Geometry check sheet. Reference: the model listing, model coordinates, mm. A direction names the side the tool comes from. Give positions to 0.01 mm unless a question says otherwise; leave off trailing zeros. Order: outer loops, then holes, each group sorted by start corner. A loop starts at its lowest first (then second) coordinate and runs counter-clockwise, first axis right, second up. Notation, with made-up numbers: M 51.5,30 L 78.5,30 A19 ccw 78.5,58 Z; hole C -25,6 d6. An arc over 180 degrees is marked long. Put each result on its own line as item: value. Start each with the question number.
Q1. Section check B-B on z = 16. Record the cut outline in (x, y).
Q2. Go/stop test with flat-tipped pins: pin 1 (7 mm diameter, centred on x = -13.5, y = 13, fed in from -Z); pin 2 (3.5 mm diameter, centred on y = 2, z = 36, fed in from -X); pin 3 (8 mm diameter, centred on y = 8, z = 33.5, fed in from +X); pin 4 (3.5 mm diameter, centred on x = 14, y = 2.5, fed in from +Z). Record where each tip stops, or that it passes through.
Q3. Material ranges on L1, parallel to X at y = 13.75, z = 18; L2, parallel to X at y = 2.5, z = 0; L3, parallel to Y at x = -19.76, z = 36.15, recorded low to high.
Q4. Access from +Z, -Z, +X, -X, +Y, -Y to the whole of each face (thin tool, end or side, straight path). Record for faces 1 (the flat face through (-25, 10, 15)), 2 (the flat face through (28, 3, 3)), 3 (the flat face through (45.296, 10.972, 37.535)), 4 (the flat face through (49, 11, 35)).
Q5. Section check A-A on x = 14. Record the cut outline in (y, z).
Q6. Section check C-C on z = -8.5. Record the cut outline in (x, y), then the cut area to 3 significant figures.
Q7. Section check D-D on y = 3.5. Record the cut outline in (x, z), then the cut area to 3 significant figures.
Q8. Mould release check, pull along Z, two halves, no side actions. Record for faces 5 (the cylindrical face through (-2.85, 3.45, 11.99)), 6 (the cylindrical face through (24.956, 3.451, -1.438)), 7 (the cylindrical face through (33.82, 3.45, 25.01)): +Z half, -Z half, draft (parallel to the pull), parting line (faces both ways), or undercut.
```python
from build123d import *

# Parameters (mm, degrees)
SKETCH1_R           = 11.05
BOSS_EXTRUDE1_DEPTH = 7
SKETCH2_R           = 1.25
BOSS_EXTRUDE2_DEPTH = 5
BOSS_EXTRUDE3_DEPTH = 20
FILLET1_R           = 10
SKETCH5_W           = 45.333333334
SKETCH5_H           = 18
CUT_EXTRUDE2_DEPTH  = 7
FILLET2_R           = 10


with BuildPart() as part:
    # Sketch1 → Boss-Extrude1 (new body)
    with BuildSketch(Plane(origin=(0, 0, 0), x_dir=(1, 0, 0), z_dir=(0, 1, 0))):
        with BuildLine():
            Line((0, 0), (0, -40))
            Line((0, -40), (28, -40))
            Line((28, -40), (28, 0))
            ThreePointArc((28, 0), (14, 14), (0, 0))
        make_face()
        with Locations(Location((14, 0, 0), (0, 0, 270))):
            Circle(SKETCH1_R, mode=Mode.SUBTRACT)
    extrude(amount=BOSS_EXTRUDE1_DEPTH)

    # Sketch2 → Boss-Extrude2 (add)
    with BuildSketch(Plane.XY.offset(40)):
        Polygon((52, 16), (52, 25), (59, 25), (59, 0), (28, 0), (28, 7), (40, 7), align=None)
        with Locations((47.76, 10.18)):
            Circle(SKETCH2_R, mode=Mode.SUBTRACT)
    boss_extrude2 = extrude(amount=-BOSS_EXTRUDE2_DEPTH)

    # Sketch3 → Boss-Extrude3 (add)
    with BuildSketch(Plane(origin=(0, 0, 35), x_dir=(-1, 0, 0), z_dir=(0, 0, -1))):
        Polygon((-52, 16), (-52, 7), (-40, 7), (-28, 7), (-28, 0), (-59, 0), (-59, 25), (-52, 25), align=None)
    boss_extrude3 = extrude(amount=BOSS_EXTRUDE3_DEPTH)

    # Mirror1: Boss-Extrude2, Boss-Extrude3 across plane
    add(boss_extrude2.mirror(Plane(origin=(14, 0, 0), x_dir=(0, 0, 1), z_dir=(1, 0, 0))))
    add(boss_extrude3.mirror(Plane(origin=(14, 0, 0), x_dir=(0, 0, 1), z_dir=(1, 0, 0))))

    # Fillet1
    fillet1_edges = [part.edges().sort_by_distance(p)[0] for p in [
        (52, 16, 37.5),
        (59, 0, 27.5),
        (40, 7, 37.5),
        (28, 3.5, 15),
        (-24, 16, 37.5),
        (-12, 7, 37.5),
        (-31, 0, 27.5),
        (0, 3.5, 15),
    ]]
    fillet(fillet1_edges, radius=FILLET1_R)

    # Sketch5 → Cut-Extrude2 (cut)
    with BuildSketch(Plane(origin=(0, 7, 0), x_dir=(1, 0, 0), z_dir=(0, 1, 0))):
        with Locations((14, -31)):
            Rectangle(SKETCH5_W, SKETCH5_H)
    extrude(amount=-CUT_EXTRUDE2_DEPTH, mode=Mode.SUBTRACT)

    # Fillet2
    fillet2_edges = [part.edges().sort_by_distance(p)[0] for p in [
        (-8.666666667, 3.5, 22),
        (36.666666667, 3.5, 22),
    ]]
    fillet(fillet2_edges, radius=FILLET2_R)


solid = part.part
```
Results found:
1. outline: M -31,10 A10 ccw -21,0 L 49,0 A10 ccw 59,10 L 59,25 L 52,25 L 52,7 L -24,7 L -24,25 L -31,25 Z
2. pin 1: passes through
2. pin 2: stops at x = -28.81
2. pin 3: stops at x = 59
2. pin 4: stops at z = 22
3. L1: x = -31 to -24, 52 to 59
3. L2: x = 0 to 2.95, 25.05 to 28
3. L3: y = 0 to 8.93, 11.43 to 12.82
4. face 1: -Z, -X, +Y, -Y
4. face 2: -Z, +X, +Y, -Y
4. face 3: +Z, -Z, +Y
4. face 4: -Z, +Y
5. outline: M 0,-14 L 7,-14 L 7,-11.05 L 0,-11.05 Z; M 0,11.05 L 7,11.05 L 7,22 L 0,22 Z
6. outline: M 2.88,0 L 6.94,0 L 6.94,7 L 2.88,7 Z; M 21.06,0 L 25.12,0 L 25.12,7 L 21.06,7 Z
6. area: 56.9 mm^2
7. outline: M -28.6,15 L -10,15 A10 cw 0,5 L 0,0 A14 ccw 28,0 L 28,5 A10 cw 38,15 L 56.6,15 L 56.6,40 L 36.67,40 L 36.67,32 A10 cw 26.67,22 L 1.33,22 A10 cw -8.67,32 L -8.67,40 L -28.6,40 Z; hole C 14,0 d22.1
7. area: 1,740 mm^2
8. face 5: -Z half
8. face 6: undercut
8. face 7: +Z half
